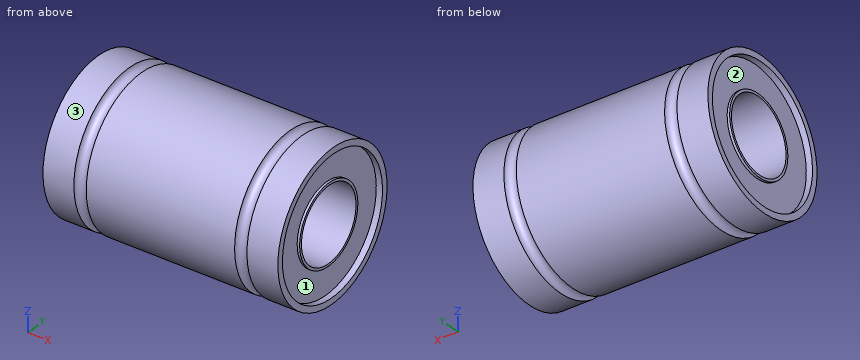
```python
from build123d import *


with BuildPart() as part:
    # Sketch1 → Revolve3 (revolve)
    with BuildSketch(Plane.XY, mode=Mode.PRIVATE) as revolve3_sk:
        with BuildLine():
            Line((3.5, 6), (15.5, 6))
            ThreePointArc((15.5, 6), (16, 5.5), (16.5, 6))
            Line((16.5, 6), (19, 6))
            Line((19, 6), (19, 5.5))
            Line((19, 5.5), (18.5, 5.5))
            Line((18.5, 5.5), (18.5, 3.2))
            Line((18.5, 3.2), (18.7, 3.2))
            Line((18.7, 3.2), (18.7, 3))
            Line((18.7, 3), (0.3, 3))
            Line((0.3, 3), (0.3, 3.2))
            Line((0.3, 3.2), (0.5, 3.2))
            Line((0.5, 3.2), (0.5, 5.5))
            Line((0.5, 5.5), (0, 5.5))
            Line((0, 5.5), (0, 6))
            Line((0, 6), (2.5, 6))
            ThreePointArc((2.5, 6), (3, 5.5), (3.5, 6))
        make_face()
    revolve(revolve3_sk.sketch.rotate(Axis((-0.95, 0, 0), (1, 0, 0)), 90), axis=Axis((-0.95, 0, 0), (1, 0, 0)))


solid = part.part
```
Source: CAD feature listing. Evaluate the final solid. Frame: model axes, mm. Face numbers are marked on the shaded views. Coordinates: 2 decimals unless noted, no trailing zeros. Write each loop counter-clockwise with the first axis right and the second up, starting at its lowest first coordinate (ties: lowest second). Pieces come first, ordered by that corner, then holes. Notation, with made-up numbers: (26, 9) -> (34, 9) arc R18 ccw to (34, 24) -> close; hole circle Ø2 at (88.25, 8). An arc over 180 degrees is marked (long way). Return JSON: item names as keys, results as strings. Group by question number.
1) Ray query, line 1 along Y through (x, z) = (18.9, 0); line 2 along Y through (x, z) = (13, -2.5); line 3 along X through (y, z) = (4.75, 2.25). Return the intervals inside material, ascending.
2) Section query D-D, the plane x = 15. Return loops of the section in (y, z).
3) Mould query, pull axis Y, two halves, no side actions, for the marked faces 1, 2 and 3. Classes: +Y half, -Y half, draft (parallel to the pull), parting line (faces both ways), or undercut.
4) Contact query for flat-ended pins moving along their axis: P1, Ø1, axis at y = 3.5, z = -3, coming from the +X side; P2, Ø7, axis at y = -1, z = 0, coming from the +X side; P3, Ø1, axis at x = 16.5, y = 2, coming from the -Z side; P4, Ø5.5, axis at y = 0, z = 0, coming from the +X side. Output: stop coordinate, or through.
5) Section query C-C, the plane x = 3. Return loops of the section in (y, z), plus the area to 3 significant figures.
From the geometry:
{
 "1": {"line 1": "-6 to -5.5, 5.5 to 6", "line 2": "-5.45 to -1.66, 1.66 to 5.45", "line 3": "0.5 to 18.5"},
 "2": {"outline": "circle Ø12 at (0, 0); hole circle Ø6 at (0, 0)"},
 "3": {"face 1": "undercut", "face 2": "undercut", "face 3": "parting line"},
 "4": {"P1": "x = 18.5", "P2": "x = 18.7", "P3": "z = -5.81", "P4": "through"},
 "5": {"outline": "circle Ø11 at (0, 0); hole circle Ø6 at (0, 0)", "area": "66.8 mm²"}
}
